The model under review builds one solid part; all positions refer to its coordinate system, in mm. A direction names the side the tool comes from. Coordinates: 2 decimals unless noted, no trailing zeros. Order: outer loops, then holes, each group sorted by start corner. A loop starts at its lowest first (then second) coordinate and runs counter-clockwise, first axis right, second up. Notation, with made-up numbers: M 11,-3 L 67,-3 A10 cw 67,15 Z; hole C 15,31.25 d11. An arc over 180 degrees is marked long. One line per item, written item: value.
Autodesk Inventor part; units mm, degrees
ref_plane "YZ Plane" through (0, 0, 0) normal (1, 0, 0) x (0, 1, 0)
ref_plane "XZ Plane" through (0, 0, 0) normal (0, 1, 0) x (-1, 0, 0)
ref_plane "XY Plane" through (0, 0, 0) normal (0, 0, 1) x (1, 0, 0)
sketch "Skizze1" plane through (0, 0, 0) normal (0, 1, 0) x (-1, 0, 0)
  line L0 (26.173, -23.607) -> (1.6422, -23.607)
  line L1 (1.6422, -23.607) -> (1.6422, -93.607)
  line L2 (1.6422, -93.607) -> (26.173, -93.607)
  line L3 (26.173, -93.607) -> (26.173, -23.607)
  line L4 (23.173, -28.607) -> (6.6422, -28.607)
  line L5 (6.6422, -28.607) -> (6.6422, -88.607)
  line L6 (6.6422, -88.607) -> (23.173, -88.607)
  line L7 (23.173, -88.607) -> (23.173, -28.607)
  point P0 (0, 0)
  dimension "d0" = 70
  dimension "d1" = 60
  dimension "d2" = 5
  dimension "d3" = 5
  dimension "d4" = 3
extrude "Extrusion1" add sketch "Skizze1" along normal blind 7
extrude "Extrusion2" add sketch "Skizze1" along normal blind 10 contours L7 L6 L5 L4
properties part number "LCD-Display"
(1) We need section A-A, the plane z = -39. State the section outline as (x, y) points.
Geometry results:
outline: M -26.17,0 L -1.64,0 L -1.64,7 L -6.64,7 L -6.64,10 L -23.17,10 L -23.17,7 L -26.17,7 Z
(2) Insertion check: pin 1 Ø1.5 at (x, y) = (-16, 8.5) entering from -Z; pin 2 Ø0.9 at (x, y) = (-18.5, 8.5) entering from +Z; pin 3 Ø0.9 at (y, z) = (8, -49) entering from +X. Each pin has a flat end and moves straight along its axis. Give the tip position at first contact, or say it passes through.
Geometry results:
pin 1: stops at z = -88.61
pin 2: stops at z = -28.61
pin 3: stops at x = -6.64
(3) For L1, parallel to X at y = 8.75, z = -42; L2, parallel to Y at x = -24, z = -73; L3, parallel to Z at x = -16, y = 9, list the stretches that pass through material, from the lowest coordinate up.
Geometry results:
L1: x = -23.17 to -6.64
L2: y = 0 to 7
L3: z = -88.61 to -28.61
(4) We need section B-B, the plane x = -21. State the section outline as (y, z) points.
Geometry results:
outline: M 0,-93.61 L 7,-93.61 L 7,-88.61 L 10,-88.61 L 10,-28.61 L 7,-28.61 L 7,-23.61 L 0,-23.61 Z
(5) Tool access review of faces 1 (the flat face through (-23.173, 8, -59)), 2 (the flat face through (-15, 8, -28.607)), 3 (the flat face through (-15, 8, -88.607)), 4 (the flat face through (-6.642, 8, -58)): name each direction out of +Z, -Z, +X, -X, +Y, -Y from which nothing blocks a thin tool from reaching the whole face with its end or side.
Geometry results:
face 1: +Z, -Z, -X, +Y
face 2: +Z, +X, -X, +Y
face 3: -Z, +X, -X, +Y
face 4: +Z, -Z, +X, +Y
(6) We need section C-C, the plane y = 8.5. State the section outline as (x, z) points, plus the area to 3 significant figures.
Geometry results:
outline: M -23.17,-88.61 L -6.64,-88.61 L -6.64,-28.61 L -23.17,-28.61 Z
area: 992 mm2
